```python
from build123d import *

# Parameters (mm, degrees)
SKETCH2_W               = 88.9
SKETCH2_H               = 152.4
BOSS_EXTRUDE1_DEPTH     = 5.9944
SKETCH4_R               = 2.7305
CUT_EXTRUDE2_DEPTH      = 1
CUT_EXTRUDE2_DEPTH_BACK = 6.9944
BOSS_EXTRUDE3_DEPTH     = 20.32
FILLET3_R               = 3.81
FILLET6_R               = 3.81
SKETCH7_W               = 2.54
SKETCH7_H               = 152.4
CUT_EXTRUDE3_DEPTH      = 18.145
CUT_EXTRUDE3_DEPTH_BACK = 6.9944
SKETCH8_W               = 86.36
SKETCH8_H               = 152.4
SKETCH8_R               = 2.7305
CUT_EXTRUDE5_DEPTH      = 5.9944
SKETCH9_R               = 2.7305
CUT_EXTRUDE6_DEPTH      = 4.064


with BuildPart() as part:
    # Sketch2 → Boss-Extrude1 (new body)
    with BuildSketch(Plane(origin=(0, 0, 0), x_dir=(1, 0, 0), z_dir=(0, 1, 0))):
        with Locations((44.45, 76.2)):
            Rectangle(SKETCH2_W, SKETCH2_H)
    extrude(amount=BOSS_EXTRUDE1_DEPTH)

    # Sketch4 → Cut-Extrude2 (cut, two sides)
    with BuildSketch(Plane(origin=(0, 5.9944, 0), x_dir=(1, 0, 0), z_dir=(0, 1, 0))) as cut_extrude2_sk:
        with Locations((45.72, 109.871331367)):
            Circle(SKETCH4_R)
        with Locations((45.72, 33.671331367)):
            Circle(SKETCH4_R)
    extrude(amount=CUT_EXTRUDE2_DEPTH, mode=Mode.SUBTRACT)
    extrude(cut_extrude2_sk.sketch, amount=-CUT_EXTRUDE2_DEPTH_BACK, mode=Mode.SUBTRACT)

    # Sketch6 → Boss-Extrude3 (add, symmetric)
    with BuildSketch(Plane.ZY.offset(-44.45)):
        Polygon((-149.86, 5.9944), (-79.121, 5.9944), (-79.121, 23.1394), (-86.106, 23.1394), (-86.106, 18.0594), (-84.201, 18.0594), (-84.201, 16.1544), (-86.106, 16.1544), (-86.106, 11.0744), (-142.875, 11.0744), (-142.875, 16.1544), (-144.78, 16.1544), (-144.78, 18.0594), (-142.875, 18.0594), (-142.875, 23.1394), (-149.86, 23.1394), align=None)
    extrude(amount=BOSS_EXTRUDE3_DEPTH, both=True)

    # Fillet3
    fillet3_edges = [part.edges().sort_by_distance(p)[0] for p in [
        (44.45, 23.1394, -149.86),
        (44.45, 23.1394, -79.121),
    ]]
    fillet(fillet3_edges, radius=FILLET3_R)

    # Fillet6
    fillet6_edges = [part.edges().sort_by_distance(p)[0] for p in [
        (24.13, 12.6619, -149.86),
        (64.77, 12.6619, -79.121),
        (24.13, 23.1394, -84.5185),
        (24.13, 12.6619, -79.121),
        (64.77, 23.1394, -84.5185),
        (64.77, 12.6619, -149.86),
        (64.77, 23.1394, -144.4625),
        (64.77, 22.023476836, -148.744076836),
        (64.77, 22.023476836, -80.236923164),
        (24.13, 23.1394, -144.4625),
        (24.13, 22.023476836, -148.744076836),
        (24.13, 22.023476836, -80.236923164),
    ]]
    fillet(fillet6_edges, radius=FILLET6_R)

    # Sketch7 → Cut-Extrude3 (cut, two sides)
    with BuildSketch(Plane(origin=(0, 5.9944, 0), x_dir=(1, 0, 0), z_dir=(0, 1, 0))) as cut_extrude3_sk:
        with Locations((1.27, 76.2)):
            Rectangle(SKETCH7_W, SKETCH7_H)
    extrude(amount=CUT_EXTRUDE3_DEPTH, mode=Mode.SUBTRACT)
    extrude(cut_extrude3_sk.sketch, amount=-CUT_EXTRUDE3_DEPTH_BACK, mode=Mode.SUBTRACT)

    # Sketch8 → Cut-Extrude5 (cut)
    with BuildSketch(Plane.XZ):
        with Locations((45.72, -76.2)):
            Rectangle(SKETCH8_W, SKETCH8_H)
        with Locations((45.72, -33.671331367)):
            Circle(SKETCH8_R, mode=Mode.SUBTRACT)
        with Locations((45.72, -109.871331367)):
            Circle(SKETCH8_R, mode=Mode.SUBTRACT)
    extrude(amount=-CUT_EXTRUDE5_DEPTH, mode=Mode.SUBTRACT)

    # Sketch9 → Cut-Extrude6 (cut)
    with BuildSketch(Plane.XZ.offset(-5.9944)):
        with Locations((44.45, -89.0905)):
            Circle(SKETCH9_R)
        with Locations((44.45, -139.8905)):
            Circle(SKETCH9_R)
    extrude(amount=-CUT_EXTRUDE6_DEPTH, mode=Mode.SUBTRACT)


solid = part.part
```
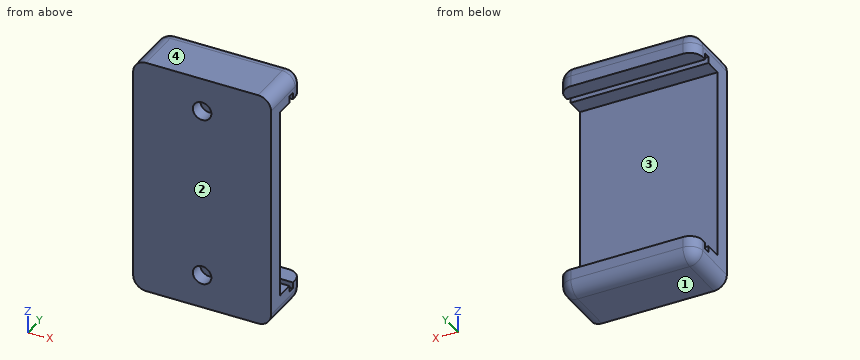
The listing builds one solid part. Answer for the finished solid, in the listing's coordinates (mm). Face numbers are marked on the shaded views. Give positions to 0.01 mm unless a question says otherwise; leave off trailing zeros. Write each loop counter-clockwise with the first axis right and the second up, starting at its lowest first coordinate (ties: lowest second). Pieces come first, ordered by that corner, then holes. Notation, with made-up numbers: (37, 73.5) -> (73, 73.5) arc R27 cw to (73, 94.5) -> close; hole circle Ø8 at (-15.75, -8.75). An arc over 180 degrees is marked (long way). Write item = value, one per line. Start each with the question number.
1) The part is cut by section B-B, the plane x = 44.45. Determine the outline of the cut face in (y, z) (3 decimals).
2) The part is cut by section C-C, the plane y = 7.75. Determine the outline of the cut face in (x, z), and give its area (3 significant figures).
3) Straight lines are drawn through the part: line 1 along Z through (x, y) = (44.45, 6.95); line 2 along Z through (x, y) = (36.5, 16.25); line 3 along Z through (x, y) = (46, 19.25) (3 decimals). For each, find the intervals that lie inside material, in ascending order.
4) The part is cut by section D-D, the plane x = 57.5. Determine the outline of the cut face in (y, z) (3 decimals).
5) Each of these flat-tipped pins is pushed along its axis until it touches: pin 1 (6 mm diameter, centred on y = 16.5, z = -136, fed in from +X); pin 2 (2.5 mm diameter, centred on x = 45, z = -139, fed in from -Y). Where does it stop, or does it pass through?
6) The part is cut by section A-A, the plane y = 12.5. Determine the outline of the cut face in (x, z) (3 decimals), and give its area (3 significant figures).
7) Determine the mould class of the marked faces 1, 2, 3 and 4 for opening direction Z: +Z half, -Z half, draft (parallel to the pull), parting line (faces both ways), or undercut.
Solutions:
q1.outline = (5.994, -149.86) -> (19.329, -149.86) arc R3.81 ccw to (23.139, -146.05) -> (23.139, -142.875) -> (18.059, -142.875) -> (18.059, -144.78) -> (16.154, -144.78) -> (16.154, -142.875) -> (11.074, -142.875) -> (11.074, -86.106) -> (16.154, -86.106) -> (16.154, -84.201) -> (18.059, -84.201) -> (18.059, -86.106) -> (23.139, -86.106) -> (23.139, -82.931) arc R3.81 ccw to (19.329, -79.121) -> (5.994, -79.121) -> (5.994, -86.36) -> (10.058, -86.36) -> (10.058, -91.821) -> (5.994, -91.821) -> (5.994, -137.16) -> (10.058, -137.16) -> (10.058, -142.621) -> (5.994, -142.621) -> close
q2.outline = (24.13, -146.05) arc R3.81 ccw to (27.94, -149.86) -> (60.96, -149.86) arc R3.81 ccw to (64.77, -146.05) -> (64.77, -82.93) arc R3.81 ccw to (60.96, -79.12) -> (27.94, -79.12) arc R3.81 ccw to (24.13, -82.93) -> close; hole circle Ø5.46 at (44.45, -139.89); hole circle Ø5.46 at (44.45, -89.09)
q2.area = 2,820 mm²
q3.line_1 = -149.86 to -142.62, -137.16 to -91.82, -86.36 to -79.12
q3.line_2 = -149.86 to -144.78, -84.2 to -79.12
q3.line_3 = -149.86 to -142.875, -86.106 to -79.121
q4.outline = (5.994, -149.86) -> (19.329, -149.86) arc R3.81 ccw to (23.139, -146.05) -> (23.139, -142.875) -> (18.059, -142.875) -> (18.059, -144.78) -> (16.154, -144.78) -> (16.154, -142.875) -> (11.074, -142.875) -> (11.074, -86.106) -> (16.154, -86.106) -> (16.154, -84.201) -> (18.059, -84.201) -> (18.059, -86.106) -> (23.139, -86.106) -> (23.139, -82.931) arc R3.81 ccw to (19.329, -79.121) -> (5.994, -79.121) -> close
q5.pin_1 = through
q5.pin_2 = 10.06
q6.outline = (24.13, -146.05) arc R3.81 ccw to (27.94, -149.86) -> (60.96, -149.86) arc R3.81 ccw to (64.77, -146.05) -> (64.77, -142.875) -> (24.13, -142.875) -> close; (24.13, -86.106) -> (64.77, -86.106) -> (64.77, -82.931) arc R3.81 ccw to (60.96, -79.121) -> (27.94, -79.121) arc R3.81 ccw to (24.13, -82.931) -> close
q6.area = 555 mm²
q7.face_1 = -Z half
q7.face_2 = draft
q7.face_3 = undercut
q7.face_4 = +Z half
